Could you check a few things on this model? Use its own coordinates, in mm. Round coordinates to 2 decimals unless told otherwise and drop trailing zeros. Loops run counter-clockwise (first coordinate to the right, second up) from the corner with the lowest first, then second, coordinate; pieces in that order, holes last.
from build123d import *

# Parameters (mm, degrees)
F0_W     = 202.830822
F0_H     = 134.983119
F1_DEPTH = 40.894
F2_R     = 35.284154
F3_DEPTH = 134.62
F5_DEPTH = 96.012


with BuildPart() as f1:
    # F0 (on Top) → F1 (new body)
    with BuildSketch(Plane.XY):
        with Locations((-54.840356, -12.115913)):
            Rectangle(F0_W, F0_H)
    extrude(amount=F1_DEPTH)

    # F2 (on face) → F3 (join)
    with BuildSketch(Plane.XY.offset(40.894)):
        with Locations((-39.066195, -9.414996)):
            Circle(F2_R)
    extrude(amount=F3_DEPTH)

    # F4 (on Front) → F5 (cut, symmetric)
    with BuildSketch(Plane.XZ):
        Polygon((38.168721, 193.453133), (-104.439028, 188.224182), (38.168721, 127.853572), align=None)
    extrude(amount=F5_DEPTH, both=True, mode=Mode.SUBTRACT)


solid = f1.part
Item 1: If we section it at A-A, the plane y = -24.5: Please give me the cut outline in (x, z), then the cut area to 3 significant figures.
Results list:
outline: (-156.26, 0) - (46.58, 0) - (46.58, 40.89) - (-7.17, 40.89) - (-7.17, 147.05) - (-70.96, 174.05) - (-70.96, 40.89) - (-156.26, 40.89) - close
area: 15,900 mm2
Item 2: If we section it at D-D, the plane y = 32: Please give me the cut outline in (x, z).
Results list:
outline: (-156.26, 0) - (46.58, 0) - (46.58, 40.89) - (-156.26, 40.89) - close
Item 3: If we section it at B-B, the plane x = -28.5: Please give me the cut outline in (y, z), then the cut area to 3 significant figures.
Results list:
outline: (-79.61, 0) - (55.38, 0) - (55.38, 40.89) - (24.25, 40.89) - (24.25, 156.08) - (-43.08, 156.08) - (-43.08, 40.89) - (-79.61, 40.89) - close
area: 13,300 mm2
Item 4: If we section it at C-C, the plane z = 113: Please give me the cut outline in (x, y) (3 decimals), then the cut area to 3 significant figures.
Results list:
outline: circle Ø70.568 at (-39.066, -9.415)
area: 3,910 mm2
Item 5: Will these pins go through, and if not, where does the flat tip stop? pin 1 (5 mm diameter, centred on x = -91.5, y = 17.5, fed in from -Z); pin 2 (6 mm diameter, centred on x = -51, y = 35, fed in from +Z).
Results list:
pin 1: stops at z = 0
pin 2: stops at z = 40.89
Item 6: If I drill on line 1 along X through (y, z) = (-9.5, 96); line 2 along Z through (x, y) = (-127.5, -16.5); line 3 along X through (y, z) = (-28, 78.5), over which ranges is the centre line in solid material (lowest first)?
Results list:
line 1: x = -74.35 to -3.78
line 2: z = 0 to 40.89
line 3: x = -69.06 to -9.07
Item 7: We'd pull the mould along X, two halves only. Please class faces 1 (the cylindrical face through (-74.316, -7.864, 107.553)), 2 (the flat face through (-56, -11, 0)), 3 (the flat face through (-156.256, -13, 20)): released by +X, released by -X, zero draft, split by the parting line, or undercut.
Results list:
face 1: split by the parting line
face 2: zero draft
face 3: released by -X
